Could you check a few things on this model? Use its own coordinates, in mm. Give positions to 0.01 mm unless a question says otherwise; leave off trailing zeros. Order: outer loops, then holes, each group sorted by start corner. A loop starts at its lowest first (then second) coordinate and runs counter-clockwise, first axis right, second up.
(1) If I drill on probe 1 along Z at (x, y) = (0, -0.7); probe 2 along X at (y, z) = (-2.3, 33); probe 3 along X at (y, z) = (-2.1, -22), over which ranges is the centre line in solid material (lowest first)?
(2) If we mould it in two halves opening along Z, with no side actions, what happens to faces 1 (the flat face through (18, -5, 7)), 2 (the cylindrical face through (16.63, -2.46, 36.31)), 3 (the flat face through (18, -2, 38.957))? For each: released by +Z, released by -Z, zero draft, split by the parting line, or undercut.
(3) Imagine slicing it at A-A, the plane x = 0. Write out the boundary of the cut face in (y, z), then the cut area to 3 significant figures.
(4) Imagine slicing it at B-B, the plane z = 0. Write out the boundary of the cut face in (x, y).
(5) Imagine slicing it at C-C, the plane y = -4.15. Write out the boundary of the cut face in (x, z) (3 decimals), then the cut area to 3 significant figures.
(6) Will this pin go through, and if not, where does the flat tip stop? pin 1 (5 mm diameter, centred on x = 5.5, z = 27, fed in from +Y).
from build123d import *

# Parameters (mm, degrees)
F2_W     = 88
F2_H     = 65
F2_R     = 2.375
F2_R_2   = 2.5
F3_DEPTH = 5


with BuildPart() as f3:
    # F2 (on Front) → F3 (new body)
    with BuildSketch(Plane.XZ):
        with Locations((18.163575, 6.457009)):
            Rectangle(F2_W, F2_H)
        with Locations((-21.928577, -21.042991)):
            Circle(F2_R, mode=Mode.SUBTRACT)
        Circle(F2_R_2, mode=Mode.SUBTRACT)
        with Locations((57.163575, -21.042991)):
            Circle(F2_R, mode=Mode.SUBTRACT)
        with Locations((-20.836425, 33.957009)):
            Circle(F2_R, mode=Mode.SUBTRACT)
        with Locations((16.940257, 25.957009)):
            Circle(F2_R, mode=Mode.SUBTRACT)
        with Locations((16.940257, 33.957009)):
            Circle(F2_R, mode=Mode.SUBTRACT)
        with Locations((56.248803, 33.957009)):
            Circle(F2_R, mode=Mode.SUBTRACT)
    extrude(amount=F3_DEPTH)


solid = f3.part
Answer block:
1. probe 1: z = -26.04 to -2.5, 2.5 to 38.96
1. probe 2: x = -25.84 to -23.01, -18.66 to 14.77, 19.11 to 54.08, 58.42 to 62.16
1. probe 3: x = -25.84 to -24.1, -19.75 to 54.99, 59.34 to 62.16
2. face 1: zero draft
2. face 2: undercut
2. face 3: released by +Z
3. outline: (-5, -26.04) - (0, -26.04) - (0, -2.5) - (-5, -2.5) - close; (-5, 2.5) - (0, 2.5) - (0, 38.96) - (-5, 38.96) - close
3. area: 300 mm2
4. outline: (-25.84, -5) - (-2.5, -5) - (-2.5, 0) - (-25.84, 0) - close; (2.5, -5) - (62.16, -5) - (62.16, 0) - (2.5, 0) - close
5. outline: (-25.836, -26.043) - (62.164, -26.043) - (62.164, 38.957) - (-25.836, 38.957) - close; hole circle Ø4.75 at (-21.929, -21.043); hole circle Ø4.75 at (-20.836, 33.957); hole circle Ø5 at (0, 0); hole circle Ø4.75 at (16.94, 25.957); hole circle Ø4.75 at (16.94, 33.957); hole circle Ø4.75 at (56.249, 33.957); hole circle Ø4.75 at (57.164, -21.043)
5. area: 5,590 mm2
6. pin 1: stops at y = 0
